from build123d import *

# Parameters (mm, degrees)
EXTRUDE3_DEPTH    = 2.54
CIRPATTERN1_COUNT = 6
FILLET4_R         = 0.127
LPATTERN1_COUNT   = 11
LPATTERN1_PITCH   = 0.4572


with BuildPart() as part:
    # Sketch1 → Revolve1 (revolve)
    with BuildSketch(Plane(origin=(0, 0, 0), x_dir=(1, 0, 0), z_dir=(0, 1, 0)), mode=Mode.PRIVATE) as revolve1_sk:
        Polygon((20.828, 2.54), (26.67, 2.54), (31.242, 0.875928089), (29.351564777, -4.318), (24.779564777, -2.653928089), (20.828, -2.653928089), align=None)
    revolve(revolve1_sk.sketch.rotate(Axis((0, 0, -37.83814433), (0, 0, 1)), 180), axis=Axis((0, 0, -37.83814433), (0, 0, 1)))  # turned: the seam where the file's is

    # Sketch3 → Extrude3 (add, symmetric)
    with BuildSketch(Plane(origin=(0, 0, 0), x_dir=(1, 0, 0), z_dir=(0, 1, 0))):
        Polygon((30.226, 1.245721847), (32.851501182, 0.290117566), (30.961065959, -4.903810522), (28.335564777, -3.948206242), align=None)
    extrude3 = extrude(amount=EXTRUDE3_DEPTH, both=True)

    # CirPattern1: Extrude3 ×6 about axis
    cirpattern1_axis = Axis((0, 0, 0), (0, 0, 1))
    for i in range(1, CIRPATTERN1_COUNT):
        add(extrude3.rotate(cirpattern1_axis, i * 360 / CIRPATTERN1_COUNT))

    # Fillet4
    fillet4_edges = [part.edges().sort_by_distance(p)[0] for p in [
        (20.828, 0, 2.653928089),
        (20.828, 0, -2.54),
    ]]
    fillet(fillet4_edges, radius=FILLET4_R)

    # Sketch4 → Cut-Revolve1 (revolve, cut)
    with BuildSketch(Plane(origin=(0, 0, 0), x_dir=(1, 0, 0), z_dir=(0, 1, 0))):
        Polygon((-20.828, -2.653928089), (-20.828, -1.774046279), (-21.59, -2.213987184), align=None)
    cut_revolve1 = revolve(axis=Axis((0, 0, -37.83814433), (0, 0, 1)), mode=Mode.SUBTRACT)

    # LPattern1: Cut-Revolve1 ×11
    with Locations(*[(0, 0, -i * LPATTERN1_PITCH) for i in range(1, LPATTERN1_COUNT)]):
        add(cut_revolve1, mode=Mode.SUBTRACT)


solid = part.part
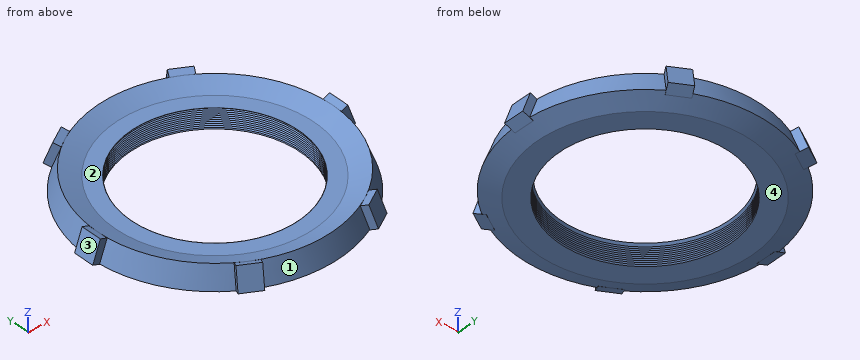
Could you check a few things on this model? Use its own coordinates, in mm. Face numbers are marked on the shaded views. Give positions to 0.01 mm unless a question says otherwise; leave off trailing zeros. Answer as CSV lines item,"result". Start each with the question number.
(1) We'd pull the mould along X, two halves only. Please class the marked faces 1, 2, 3 and 4: released by +X, released by -X, zero draft, split by the parting line, or undercut.
(2) I'm going to push flat-ended pins straight in: pin 1 Ø2 at (x, z) = (-6.5, 0) entering from +Y; pin 2 Ø4 at (y, z) = (-5.5, -1.5) entering from -X; pin 3 Ø6 at (x, y) = (18.5, 8) entering from +Z. Where does each tip first touch, or does it pass through?
(3) I need wall thicknesses on probe 1 along X at (y, z) = (5.5, 1.5); probe 2 along Z at (x, y) = (-15.5, -17.5); probe 3 along X at (y, z) = (-5, 1). Which ranges of each line are inside material? Lowest first, please.
Computed:
1,face 1,"undercut"
1,face 2,"undercut"
1,face 3,"released by -X"
1,face 4,"zero draft"
2,pin 1,"stops at y = 30.66"
2,pin 2,"stops at x = -31.03"
2,pin 3,"stops at z = 2.65"
3,probe 1,"x = -29.88 to -20.52, 20.52 to 29.88"
3,probe 2,"z = -2.54 to 2.65"
3,probe 3,"x = -30.15 to -20.72, 20.72 to 30.15"
